Autodesk Inventor part; units mm, degrees
ref_plane "YZ Plane" through (0, 0, 0) normal (1, 0, 0) x (0, 1, 0)
ref_plane "XZ Plane" through (0, 0, 0) normal (0, 1, 0) x (-1, 0, 0)
ref_plane "XY Plane" through (0, 0, 0) normal (0, 0, 1) x (1, 0, 0)
sketch "Sketch1" plane through (0, 0, 0) normal (0, 1, 0) x (-1, 0, 0)
  line L0 (6.7607, 5.7456) -> (-18.6393, 5.7456)
  line L1 (-18.6393, 5.7456) -> (-18.6393, -248.2544)
  line L2 (-18.6393, -248.2544) -> (6.7607, -248.2544)
  line L3 (6.7607, -248.2544) -> (6.7607, 5.7456)
  point P0 (0, 0)
  dimension "d0" = 25.4
  dimension "d1" = 254
extrude "Extrusion1" add sketch "Sketch1" along normal blind 25.4
sketch "Sketch2" plane through (18.6393, 0, 5.7456) normal (1, 0, 0) x (0, 0, -1)
  line L0 (0, 0) -> (0, 25.4)
  line L1 (254, 0) -> (254, 25.4)
  line L2 (0, 15.875) -> (254, 15.875)
  line L3 (254, 15.875) -> (254, 9.525)
  line L4 (254, 9.525) -> (0, 9.525)
  line L5 (0, 9.525) -> (0, 15.875)
  line L6 (0, 25.4) -> (254, 25.4)
  line L7 (0, 0) -> (254, 0)
  point P0 (5.7456, 0)
  point P1 (0, 9.525)
  dimension "d4" = 6.35
  dimension "d5" = 9.525
extrude "Extrusion2" cut sketch "Sketch2" against normal blind 6.35 contours L0 L2 L1 L4
sketch "Sketch3" plane through (-6.7607, 0, -248.2544) normal (-1, 0, 0) x (0, 0, 1)
  circle A0 centre (241.3, 12.7) radius 1.5875
  circle A1 centre (12.7, 12.7) radius 1.5875
  line L0 (0, 0) -> (0, 25.4)
  line L1 (0, 25.4) -> (254, 25.4)
  line L2 (254, 0) -> (254, 25.4)
  line L3 (0, 0) -> (254, 0)
  point P0 (248.2544, 0)
  dimension "d8" = 3.175
  dimension "d9" = 3.175
  dimension "d10" = 12.7
  dimension "d11" = 12.7
  dimension "d12" = 12.7
  dimension "d13" = 12.7
extrude "Extrusion3" cut sketch "Sketch3" against normal blind 76.2 contours A0 | A1
chamfer "Chamfer1" distance 3.175 angle 45 2 edges at (-6.7607, 12.7, -237.1419) (-6.7607, 12.7, -8.5419)
properties part number "glass holder drawr X8"
Geometry: final body of the model. Coordinates: model frame, mm. A direction names the side the tool comes from. Give positions to 0.01 mm unless a question says otherwise; leave off trailing zeros. Loops run counter-clockwise (first coordinate to the right, second up) from the corner with the lowest first, then second, coordinate; pieces in that order, holes last. Notation, with made-up numbers: (88, -31.75) -> (127, -31.75) arc R28 cw to (127, -9.75) -> close; hole circle Ø8 at (9.25, 22.25). An arc over 180 degrees is marked (long way). Put each result on its own line as item: value.
1. Cut plane A-A (z = -90). Return the cut outline in (x, y) (3 decimals).
Taken from the geometry:
outline: (-6.761, 0) -> (18.639, 0) -> (18.639, 9.525) -> (12.289, 9.525) -> (12.289, 15.875) -> (18.639, 15.875) -> (18.639, 25.4) -> (-6.761, 25.4) -> close
2. Set-up query: faces 4 (the flat face through (18.639, 21, -119)), 5 (the flat face through (16, 15.875, -119)). Return all of +Z, -Z, +X, -X, +Y, -Y with unobstructed straight access to the full face (end or side cutting, diameter ignored); none if empty.
Taken from the geometry:
face 4: +Z, -Z, +X, +Y, -Y
face 5: +Z, -Z, +X
3. Pull-direction query (Z, two-part tool) for faces 1 (the flat face through (6, 13, -248.254)), 2 (the conical face through (-3.784, 14.206, -234.594)), 3 (the flat face through (16, 9.525, -123)); classes: released by +Z, released by -Z, zero draft, split by the parting line, or undercut.
Taken from the geometry:
face 1: released by -Z
face 2: undercut
face 3: zero draft
4. Ray query, line 1 along Y through (x, z) = (16.5, -126) (3 decimals); line 2 along X through (y, z) = (14, -134). Return the intervals inside material, ascending. Write a range as [from, to].
Taken from the geometry:
line 1: y = [0, 9.525], [15.875, 25.4]
line 2: x = [-6.76, 12.29]
5. Pin query (flat end, axial travel): P1, Ø7, axis at y = 12, z = -148, coming from the +X side. Return the tip coordinate at first contact, or that it passes through.
Taken from the geometry:
P1: stops at x = 18.64
